```python
from build123d import *


with BuildPart() as part:
    # BodySke → Body (revolve)
    with BuildSketch(Plane.XY, mode=Mode.PRIVATE) as body_sk:
        Polygon((3, 8), (58, 8), (60, 7.464101615), (60, 5.25), (58.5, 5.25), (57.431902002, 3.4), (35, 3.4), (33.591673888, 0), (0, 0), (0, 7.196152423), align=None)
    revolve(body_sk.sketch.rotate(Axis((0, 0, 0), (1, 0, 0)), 90), axis=Axis((0, 0, 0), (1, 0, 0)))


solid = part.part
```
The listing builds one solid part. Answer for the finished solid, in the listing's coordinates (mm). A direction names the side the tool comes from. Give positions to 0.01 mm unless a question says otherwise; leave off trailing zeros. Order: outer loops, then holes, each group sorted by start corner. A loop starts at its lowest first (then second) coordinate and runs counter-clockwise, first axis right, second up. Notation, with made-up numbers: (-9, 32.5) - (0, 32.5) arc R32 ccw to (0, 68.5) - close; hole circle Ø6 at (23, 9). An arc over 180 degrees is marked (long way). Answer in a Markdown table with one row per item. Add a question column.
Q1. Find the intervals of material crossed by line 1 along Y through (x, z) = (32.5, 3.5); line 2 along Y through (x, z) = (49.75, 0); line 3 along Y through (x, z) = (59.6, 0), in increasing order. Write a range as [from, to].
Q2. For a pull along Z with two mould halves and no side action, classify faces 3 (the flat face through (60, -5.1, -1.8)), 4 (the conical face through (0.19, 6.43, 3.34)), 5 (the cylindrical face through (59.2, -1.6, 5)) as released by +Z, released by -Z, zero draft, split by the parting line, or undercut.
Q3. Given P1, Ø9, axis at y = 0, z = 0, coming from the -X side; P2, Ø6, axis at x = 15, z = -6.5, coming from the -Y side; P3, Ø3, axis at x = 12.5, y = 3.5, coming from the +Z side; P4, Ø4, axis at x = 39.5, y = -3, coming from the +Z side, each flat-ended and moving along its own axis, determine where each tip first touches the part or whether it passes through.
Q4. The part is cut by section A-A (x = 55.5). Determine the outline of the cut face in (y, z).
Q5. Which of the six approach directions +Z, -Z, +X, -X, +Y, -Y give full straight-line access (tool end or side, diameter ignored) to faces 1 (the cylindrical face through (30.88, 7.81, -1.73)), 2 (the cylindrical face through (46.06, 3.32, -0.74))?
Q6. The part is cut by section B-B (x = 23). Determine the outline of the cut face in (y, z), then the cut area to 3 significant figures.
Determined:
| question | item | result |
|---|---|---|
| 1 | line 1 | y = [-7.19, 7.19] |
| 1 | line 2 | y = [-8, -3.4], [3.4, 8] |
| 1 | line 3 | y = [-7.57, -5.25], [5.25, 7.57] |
| 2 | face 3 | zero draft |
| 2 | face 4 | split by the parting line |
| 2 | face 5 | undercut |
| 3 | P1 | stops at x = 0 |
| 3 | P2 | stops at y = -7.19 |
| 3 | P3 | stops at z = 7.75 |
| 3 | P4 | stops at z = 7.94 |
| 4 | outline | circle Ø16 at (0, 0); hole circle Ø6.8 at (0, 0) |
| 5 | face 1 | +X, -X |
| 5 | face 2 | +X |
| 6 | outline | circle Ø16 at (0, 0) |
| 6 | area | 201 mm² |
